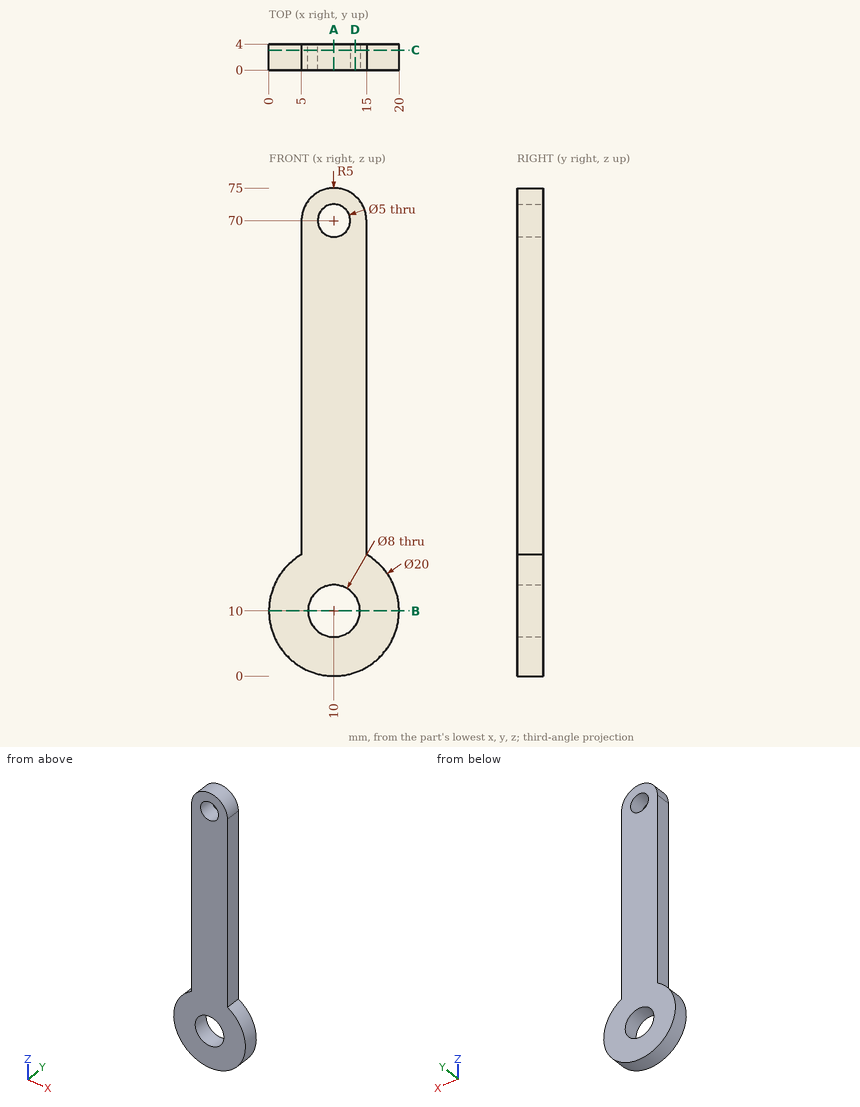
Geometry: see drawing. Coordinates: mm, zero at the bounding-box minimum. Give positions to 0.01 mm unless a question says otherwise; leave off trailing zeros. Loops run counter-clockwise (first coordinate to the right, second up) from the corner with the lowest first, then second, coordinate; pieces in that order, holes last. Notation, with made-up numbers: (83, 60.5) -> (122, 60.5) arc R29 ccw to (122, 92.5) -> close; hole circle Ø7 at (53.5, 22). An arc over 180 degrees is marked (long way). Use one line per item in the form item = value.
Item 1: Section query A-A on x = 10. Output: boundary loops of the cut face in (y, z), and give its area (3 significant figures).
A:
outline = (0, 0) -> (4, 0) -> (4, 6) -> (0, 6) -> close; (0, 14) -> (4, 14) -> (4, 67.5) -> (0, 67.5) -> close; (0, 72.5) -> (4, 72.5) -> (4, 75) -> (0, 75) -> close
area = 248 mm^2
Item 2: Pin query (flat end, axial travel): P1, Ø6.5, axis at x = 10, z = 70, coming from the +Y side; P2, Ø1.2, axis at y = 2, z = 46, coming from the +X side; P3, Ø1.5, axis at x = 16, y = 1, coming from the -Z side. Return the tip coordinate at first contact, or that it passes through.
A:
P1 = 4
P2 = 15
P3 = 1.49
Item 3: Line query: probe 1 along Z at (x, y) = (10, 2.95); probe 2 along Z at (x, y) = (8, 2.2); probe 3 along X at (y, z) = (3.4, 67). Output: solid intervals per line, ascending.
A:
probe_1 = 0 to 6, 14 to 67.5, 72.5 to 75
probe_2 = 0.2 to 6.54, 13.46 to 68.5, 71.5 to 74.58
probe_3 = 5 to 15
Item 4: Section query D-D on x = 13.25. Output: boundary loops of the cut face in (y, z), and give its area (3 significant figures).
A:
outline = (0, 0.54) -> (4, 0.54) -> (4, 7.67) -> (0, 7.67) -> close; (0, 12.33) -> (4, 12.33) -> (4, 73.8) -> (0, 73.8) -> close
area = 274 mm^2
Item 5: Section query C-C on y = 3.05. Output: boundary loops of the cut face in (x, z), and give its area (3 significant figures).
A:
outline = (5, 18.66) arc R10 ccw (long way) to (15, 18.66) -> (15, 70) arc R5 ccw to (5, 70) -> close; hole circle Ø8 at (10, 10); hole circle Ø5 at (10, 70)
area = 788 mm^2
Item 6: Section query B-B on z = 10. Output: boundary loops of the cut face in (x, y), and give its area (3 significant figures).
A:
outline = (0, 0) -> (6, 0) -> (6, 4) -> (0, 4) -> close; (14, 0) -> (20, 0) -> (20, 4) -> (14, 4) -> close
area = 48.0 mm^2
